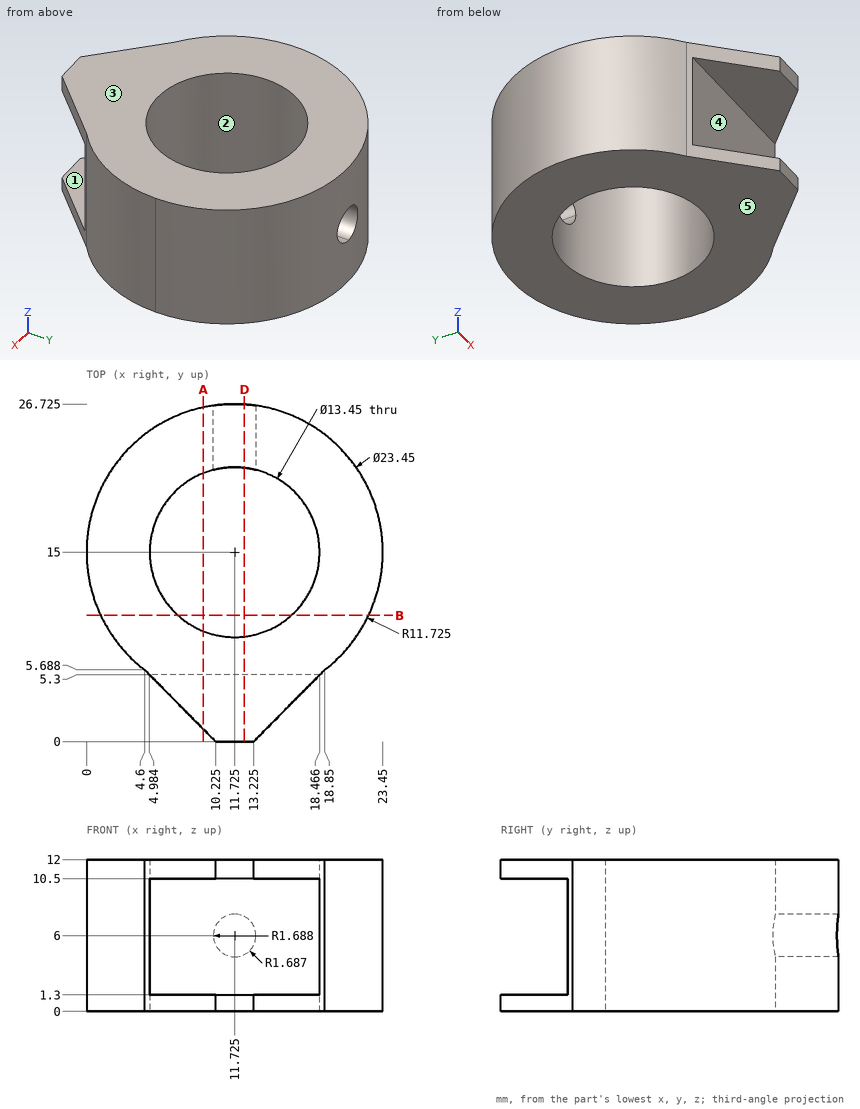
The drawing under review shows one solid part. Ordinate dimensions are in mm from its lowest x, y, z. A direction names the side the tool comes from. Round coordinates to 2 decimals unless told otherwise and drop trailing zeros. Loops run counter-clockwise (first coordinate to the right, second up) from the corner with the lowest first, then second, coordinate; pieces in that order, holes last.
Item 1: Take a section at A-A (x = 9.25). Write out the cut boundary in (y, z) (1 decimal).
Determined:
outline: (1, 0) - (8.7, 0) - (8.7, 12) - (1, 12) - (1, 10.5) - (5.3, 10.5) - (5.3, 1.3) - (1, 1.3) - close; (21.3, 0) - (26.5, 0) - (26.5, 12) - (21.3, 12) - close
Item 2: For line 1 (Y direction, x = 12, z = 9.75); line 2 (X direction, y = 19, z = 9) (1 decimal); line 3 (Y direction, x = 14.75, z = 6.5) (1 decimal), list the stretches that pass through material, from the lowest coordinate up.
Determined:
line 1: y = 5.3 to 8.28, 21.72 to 26.72
line 2: x = 0.7 to 6.3, 17.1 to 22.7
line 3: y = 5.3 to 9, 21 to 26.3
Item 3: Mouldability with a two-part tool opening along Z and no side actions: class the marked faces 3, 4 and 5 as released by +Z, released by -Z, zero draft, split by the parting line, or undercut.
Determined:
face 3: released by +Z
face 4: undercut
face 5: released by -Z
Item 4: Take a section at B-B (y = 10). Write out the cut boundary in (x, z).
Determined:
outline: (1.12, 0) - (7.23, 0) - (7.23, 12) - (1.12, 12) - close; (16.22, 0) - (22.33, 0) - (22.33, 12) - (16.22, 12) - close
Item 5: Clearance check with flat-ended pins moving along their axes: pin 1 Ø5 at (y, z) = (10, 10) entering from -X; pin 2 Ø5 at (y, z) = (3, 10) entering from +X (1 decimal); pin 3 Ø1.5 at (x, y) = (17.5, 16) entering from +Z; pin 4 Ø2 at (y, z) = (16.5, 4) entering from +X. State where each tip first meets the part, or that it passes through.
Determined:
pin 1: stops at x = 0.27
pin 2: stops at x = 18.7
pin 3: passes through
pin 4: stops at x = 23.44
Item 6: For the marked faces 1 and 2, list the 3-axis set-ups (+Z, -Z, +X, -X, +Y, -Y) from which the entire face can be reached by the end or side of a thin tool; tool diameter is ignored.
Determined:
face 1: +X, -X, -Y
face 2: +Z, -Z
Item 7: Take a section at D-D (x = 12.5). Write out the cut boundary in (y, z).
Determined:
outline: (0, 0) - (8.32, 0) - (8.32, 12) - (0, 12) - (0, 10.5) - (5.3, 10.5) - (5.3, 1.3) - (0, 1.3) - close; (21.68, 0) - (26.7, 0) - (26.7, 4.5) - (21.68, 4.5) - close; (21.68, 7.5) - (26.7, 7.5) - (26.7, 12) - (21.68, 12) - close
